The model under review builds one solid part; all positions refer to its coordinate system, in mm. Face numbers are marked on the shaded views. Round coordinates to 2 decimals unless told otherwise and drop trailing zeros. Loops run counter-clockwise (first coordinate to the right, second up) from the corner with the lowest first, then second, coordinate; pieces in that order, holes last. Notation, with made-up numbers: M 56,69.25 L 64,69.25 A22 ccw 64,96.25 Z; hole C 57.25,-15.75 d5. An arc over 180 degrees is marked long. One line per question, with ' | ' between items.
from build123d import *

# Parameters (mm, degrees)
BASPROSKE_W     = 20
BASPROSKE_H     = 26.25
TOOTHCUT_DEPTH  = 43.167819484
TEETHCUTS_COUNT = 33
TEETHCUTS_ANGLE = 349.090909091
BORSKE_R        = 15
BORE_DEPTH      = 50.0000508
KEYSKE_W        = 10
KEYSKE_H        = 18.3
KEYWAY_DEPTH    = 50.0000508
EXTRUDE_START   = 1
SKETCH_1_R      = 28
EXTRUDE_2_DEPTH = 1
SKETCH_2_R      = 28
EXTRUDE_3_DEPTH = 1
EXTRUDE_4_DEPTH = 10


with BuildPart() as part:
    # BasProSke → Base-Revolve (revolve)
    with BuildSketch(Plane(origin=(0, 0, 0), x_dir=(1, 0, 0), z_dir=(0, 1, 0)), mode=Mode.PRIVATE) as base_revolve_sk:
        with Locations((10, 13.125)):
            Rectangle(BASPROSKE_W, BASPROSKE_H)
    revolve(base_revolve_sk.sketch.rotate(Axis((-10, 0, 0), (1, 0, 0)), 180), axis=Axis((-10, 0, 0), (1, 0, 0)))

    # TooCutSke → ToothCut (cut, through all)
    with BuildSketch(Plane(origin=(0, 0, 0), x_dir=(0, 0, -1), z_dir=(1, 0, 0))):
        with BuildLine():
            ThreePointArc((0.683690741, 22.863780155), (0, 22.874), (-0.683690741, 22.863780155))
            ThreePointArc((-0.683690741, 22.863780155), (-1.217783987, 24.592276227), (-2.057504394, 26.194719331))
            ThreePointArc((-2.057504394, 26.194719331), (0, 26.2754), (2.057504394, 26.194719331))
            ThreePointArc((2.057504394, 26.194719331), (1.217783987, 24.592276227), (0.683690741, 22.863780155))
        make_face()
    toothcut = extrude(amount=TOOTHCUT_DEPTH, mode=Mode.SUBTRACT)

    # TeethCuts: ToothCut ×33 about axis
    teethcuts_axis = Axis((-10, 0, 0), (1, 0, 0))
    for i in range(1, TEETHCUTS_COUNT):
        add(toothcut.rotate(teethcuts_axis, i * TEETHCUTS_ANGLE / (TEETHCUTS_COUNT - 1)), mode=Mode.SUBTRACT)

    # BorSke → Bore (cut, symmetric)
    with BuildSketch(Plane(origin=(0, 0, 0), x_dir=(0, 0, -1), z_dir=(1, 0, 0))):
        with Locations(Location((0, 0, 0), (0, 0, 180))):
            Circle(BORSKE_R)
    extrude(amount=BORE_DEPTH, both=True, mode=Mode.SUBTRACT)

    # KeySke → Keyway (cut, symmetric)
    with BuildSketch(Plane(origin=(0, 0, 0), x_dir=(0, 0, -1), z_dir=(1, 0, 0))):
        with Locations((0, 9.15)):
            Rectangle(KEYSKE_W, KEYSKE_H)
    extrude(amount=KEYWAY_DEPTH, both=True, mode=Mode.SUBTRACT)

    # Эскиз1 → Бобышка-Вытянуть2 (add)
    with BuildSketch(Plane(origin=(20, 0, 0), x_dir=(0, 0, -1), z_dir=(1, 0, 0)).offset(EXTRUDE_START)):
        Circle(SKETCH_1_R)
        with BuildLine():
            Line((5, 18.3), (-5, 18.3))
            Line((-5, 18.3), (-5, 14.142135624))
            ThreePointArc((-5, 14.142135624), (0, -15), (5, 14.142135624))
            Line((5, 14.142135624), (5, 18.3))
        make_face(mode=Mode.SUBTRACT)
    extrude(amount=-EXTRUDE_2_DEPTH)

    # Эскиз2 → Бобышка-Вытянуть3 (add)
    with BuildSketch(Plane.ZY):
        with Locations(Location((0, 0, 0), (0, 0, 180))):
            Circle(SKETCH_2_R)
        with BuildLine():
            Line((-5, 18.3), (-5, 14.142135624))
            ThreePointArc((-5, 14.142135624), (0, -15), (5, 14.142135624))
            Line((5, 14.142135624), (5, 18.3))
            Line((5, 18.3), (-5, 18.3))
        make_face(mode=Mode.SUBTRACT)
    extrude(amount=EXTRUDE_3_DEPTH)


with BuildPart() as body_2:
    # Эскиз4 → Бобышка-Вытянуть4 (new, symmetric)
    with BuildSketch(Plane(origin=(10, 0, 0), x_dir=(0, 0, -1), z_dir=(1, 0, 0))):
        with BuildLine():
            Line((-2.057504394, 26.194719331), (2.057504394, 26.194719331))
            ThreePointArc((2.057504394, 26.194719331), (1.217783987, 24.592276227), (0.683690741, 22.863780155))
            ThreePointArc((0.683690741, 22.863780155), (0, 22.874), (-0.683690741, 22.863780155))
            ThreePointArc((-0.683690741, 22.863780155), (-1.217783987, 24.592276227), (-2.057504394, 26.194719331))
        make_face()
    extrude(amount=EXTRUDE_4_DEPTH, both=True)


solid = body_2.part
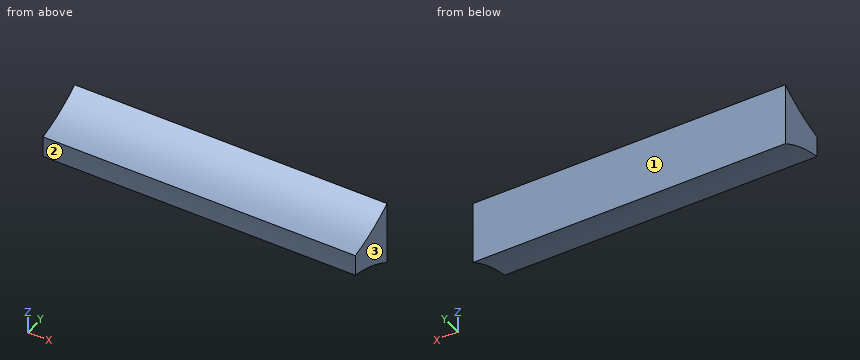
1) Insertion check: P1, Ø1, axis at x = 3, z = 0, coming from the -Y side. The pin has a flat end and moves straight along its axis. Give the tip position at first contact, or say it passes through.
Output values:
P1: stops at y = 22.87
2) For line 1 (Y direction, x = 18.5, z = 0.55); line 2 (Z direction, x = 10.5, y = 23.1); line 3 (Z direction, x = 2.25, y = 26.05), list the stretches that pass through material, from the lowest coordinate up.
Output values:
line 1: y = 22.87 to 26.19 | line 2: z = -0.74 to 0.74 | line 3: z = -1.97 to 1.97
3) Mouldability with a two-part tool opening along Y and no side actions: class the marked faces 1, 2 and 3 as +Y half, -Y half, draft (parallel to the pull), parting line (faces both ways), or undercut.
Output values:
face 1: +Y half | face 2: -Y half | face 3: draft
4) Add section B-B on z = -1. State the section outline as (x, y) points.
Output values:
outline: M 0,24.01 L 20,24.01 L 20,26.19 L 0,26.19 Z
5) Add section A-A on x = 9. State the section outline as (y, z) points.
Output values:
outline: M 22.86,-0.68 A9.9 cw 26.19,-2.06 L 26.19,2.06 A9.9 cw 22.86,0.68 A22.87 cw Z
